from build123d import *

# Parameters (mm, degrees)
SKETCH1_W           = 10
SKETCH1_H           = 25.5
BOSS_EXTRUDE1_DEPTH = 8
SKETCH2_W           = 0.5
SKETCH2_H           = 23
BOSS_EXTRUDE2_DEPTH = 3.3


with BuildPart() as part:
    # Sketch1 → Boss-Extrude1 (new body)
    with BuildSketch(Plane(origin=(0, 0, 0), x_dir=(1, 0, 0), z_dir=(0, 1, 0))):
        Rectangle(SKETCH1_W, SKETCH1_H)
    extrude(amount=-BOSS_EXTRUDE1_DEPTH)

    # Sketch2 → Boss-Extrude2 (add)
    with BuildSketch(Plane.XZ.offset(8)):
        with Locations((4, 0)):
            Rectangle(SKETCH2_W, SKETCH2_H)
        with Locations((-4, 0)):
            Rectangle(SKETCH2_W, SKETCH2_H)
    extrude(amount=BOSS_EXTRUDE2_DEPTH)


solid = part.part
Work out the finished part from the listing and answer in its coordinate system (mm). A direction names the side the tool comes from. Give positions to 0.01 mm unless a question says otherwise; leave off trailing zeros. Loops run counter-clockwise (first coordinate to the right, second up) from the corner with the lowest first, then second, coordinate; pieces in that order, holes last. Notation, with made-up numbers: (27.5, -32.75) -> (60.5, -32.75) arc R22 ccw to (60.5, -21.75) -> close; hole circle Ø5 at (-10.5, -5.75). An arc over 180 degrees is marked (long way). Use a Markdown table: item, result. Add a question column.
1. Section B-B on z = -1.5 is taken. Determine the outline of the cut face in (x, y).
2. Section C-C on x = -1.25 is taken. Determine the outline of the cut face in (y, z), and give its area (3 significant figures).
3. Determine the mould class of faces 5 (the flat face through (0, -8, 0)), 6 (the flat face through (-5, -4, 0)), 7 (the flat face through (0, 0, 0)) for opening direction X: released by +X, released by -X, zero draft, split by the parting line, or undercut.
4. Section A-A on y = -8.75 is taken. Determine the outline of the cut face in (x, z), and give its area (3 significant figures).
5. Find the intervals of material crossed by probe 1 along X at (y, z) = (-8.25, 4.25); probe 2 along Y at (x, z) = (-1, 1.25), in increasing order.
6. For faces 1 (the flat face through (-3.75, -10, 0)), 2 (the flat face through (5, -4, 0)), 3 (the flat face through (4.25, -10, 0)), 4 (the flat face through (-4.25, -10, 0)), determine the directions among +Z, -Z, +X, -X, +Y, -Y from which every point of the face is accessible in a straight line to the end or side of a thin tool.
7. Flat-ended cylindrical pins translate along their axes: pin 1 Ø1 at (y, z) = (-9, -0.5) entering from -X; pin 2 Ø1 at (y, z) = (-10, -1) entering from +X; pin 3 Ø3 at (x, z) = (-1, 1) entering from -Y. Find the tip coordinate at first contact, or state that the pin passes through.
Results below:
| question | item | result |
|---|---|---|
| 1 | outline | (-5, -8) -> (-4.25, -8) -> (-4.25, -11.3) -> (-3.75, -11.3) -> (-3.75, -8) -> (3.75, -8) -> (3.75, -11.3) -> (4.25, -11.3) -> (4.25, -8) -> (5, -8) -> (5, 0) -> (-5, 0) -> close |
| 2 | outline | (-8, -12.75) -> (0, -12.75) -> (0, 12.75) -> (-8, 12.75) -> close |
| 2 | area | 204 mm^2 |
| 3 | face 5 | undercut |
| 3 | face 6 | released by -X |
| 3 | face 7 | zero draft |
| 4 | outline | (-4.25, -11.5) -> (-3.75, -11.5) -> (-3.75, 11.5) -> (-4.25, 11.5) -> close; (3.75, -11.5) -> (4.25, -11.5) -> (4.25, 11.5) -> (3.75, 11.5) -> close |
| 4 | area | 23.0 mm^2 |
| 5 | probe 1 | x = -4.25 to -3.75, 3.75 to 4.25 |
| 5 | probe 2 | y = -8 to 0 |
| 6 | face 1 | +Z, -Z, -Y |
| 6 | face 2 | +Z, -Z, +X, +Y, -Y |
| 6 | face 3 | +Z, -Z, +X, -Y |
| 6 | face 4 | +Z, -Z, -X, -Y |
| 7 | pin 1 | stops at x = -4.25 |
| 7 | pin 2 | stops at x = 4.25 |
| 7 | pin 3 | stops at y = -8 |
